Could you check a few things on this drawing? It's one solid part, dimensions in mm from its lowest x, y, z. Round coordinates to 2 decimals unless told otherwise and drop trailing zeros. Loops run counter-clockwise (first coordinate to the right, second up) from the corner with the lowest first, then second, coordinate; pieces in that order, holes last. Notation, with made-up numbers: (31, 71) -> (90, 71) arc R19 ccw to (90, 105) -> close; hole circle Ø5 at (52.25, -40). An arc over 180 degrees is marked (long way). Use one line per item in the form item = value. Start each with the question number.
Item 1: Thinking about a two-plate mould opening in Y: for the marked faces 1 and 2, which applies, released by +Y, released by -Y, zero draft, split by the parting line, or undercut?
Item 2: If we section it at C-C (x = 44): Write out the boundary of the cut face in (y, z), then the cut area to 3 significant figures.
Item 3: If I drill on L1, parallel to Y at x = 36, z = 6.25; L2, parallel to Z at x = 2, y = 6.5 (3 decimals); L3, parallel to Z at x = 43, y = 8.75, over which ranges is the centre line in solid material (lowest first)? Write a range as [from, to].
Item 4: If we section it at A-A (z = 6.25): Write out the boundary of the cut face in (x, y), then the cut area to 3 significant figures.
Item 5: I'm going to push flat-ended pins straight in: pin 1 Ø6 at (x, y) = (36, 10.5) entering from +Z; pin 2 Ø1.5 at (x, y) = (26.5, 3.5) entering from -Z; pin 3 Ø1 at (x, y) = (19.5, 10) entering from -Z. Where does each tip first touch, or does it pass through?
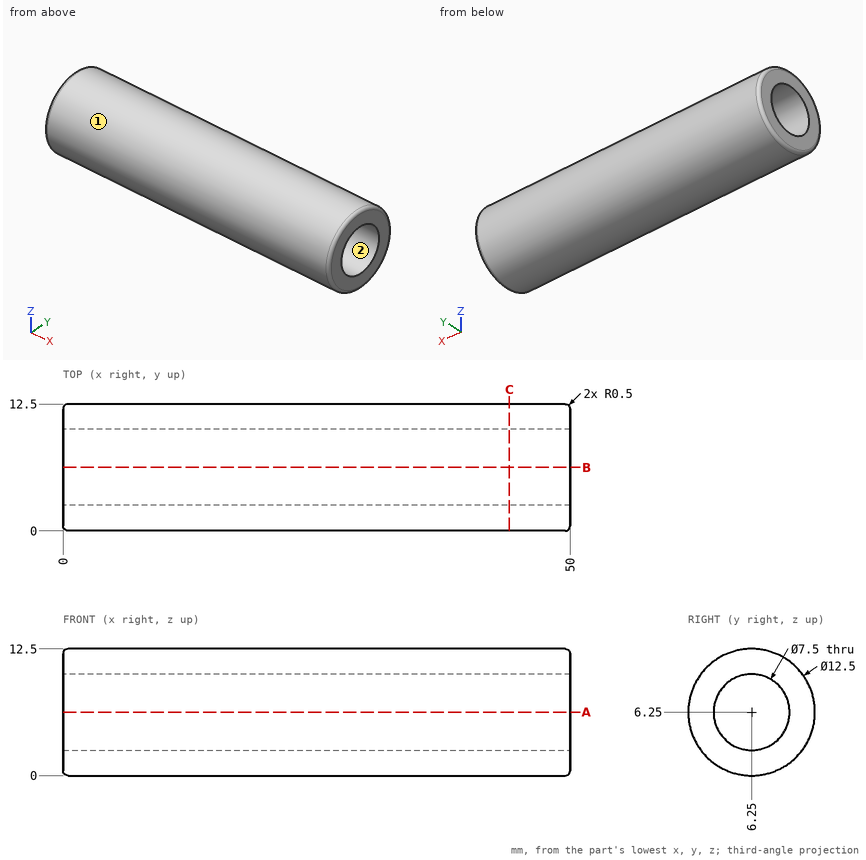
Values found:
q1.face_1 = split by the parting line
q1.face_2 = undercut
q2.outline = circle Ø12.5 at (6.25, 6.25); hole circle Ø7.5 at (6.25, 6.25)
q2.area = 78.5 mm2
q3.L1 = [0, 2.5], [10, 12.5]
q3.L2 = [0.005, 2.508], [9.992, 12.495]
q3.L3 = [0.52, 3.45], [9.05, 11.98]
q4.outline = (0, 0.5) arc R0.5 ccw to (0.5, 0) -> (49.5, 0) arc R0.5 ccw to (50, 0.5) -> (50, 2.5) -> (0, 2.5) -> close; (0, 10) -> (50, 10) -> (50, 12) arc R0.5 ccw to (49.5, 12.5) -> (0.5, 12.5) arc R0.5 ccw to (0, 12) -> close
q4.area = 250 mm2
q5.pin_1 = 12.37
q5.pin_2 = 0.33
q5.pin_3 = 0.91
